The drawing under review shows one solid part. Ordinate dimensions are in mm from its lowest x, y, z. A direction names the side the tool comes from. Give positions to 0.01 mm unless a question says otherwise; leave off trailing zeros. Write each loop counter-clockwise with the first axis right and the second up, starting at its lowest first coordinate (ties: lowest second). Pieces come first, ordered by that corner, then holes.
Q1. We need section B-B (y = 11.25). Write out the cut boundary in (x, z), then the cut area to 3 significant figures.
Q2. Insertion check: P1, Ø4, axis at x = 5, y = 8, coming from the +Z side; P2, Ø1.5, axis at x = 5.5, y = 2.5, coming from the -Z side; P3, Ø3, axis at y = 7.5, z = 4.5, coming from the +X side. Each pin has a flat end and moves straight along its axis. Give the tip position at first contact, or say it passes through.
Q3. We need section A-A (y = 1.75). Write out the cut boundary in (x, z).
Q4. For line 1 (Y direction, x = 1.5, z = 2.5); line 2 (Y direction, x = 3.5, z = 2.5); line 3 (X direction, y = 14, z = 3.25), list the stretches that pass through material, from the lowest coordinate up.
Q5. Machinability: for the marked faces 1 and 2, which of the approach directions +Z, -Z, +X, -X, +Y, -Y give a long, thin tool a straight path to every point of the face, cutting with its end or side? Answer none if there is none.
Q6. Mouldability with a two-part tool opening along Z and no side actions: class the marked faces 3, 4, 5 and 6 as released by +Z, released by -Z, zero draft, split by the parting line, or undercut.
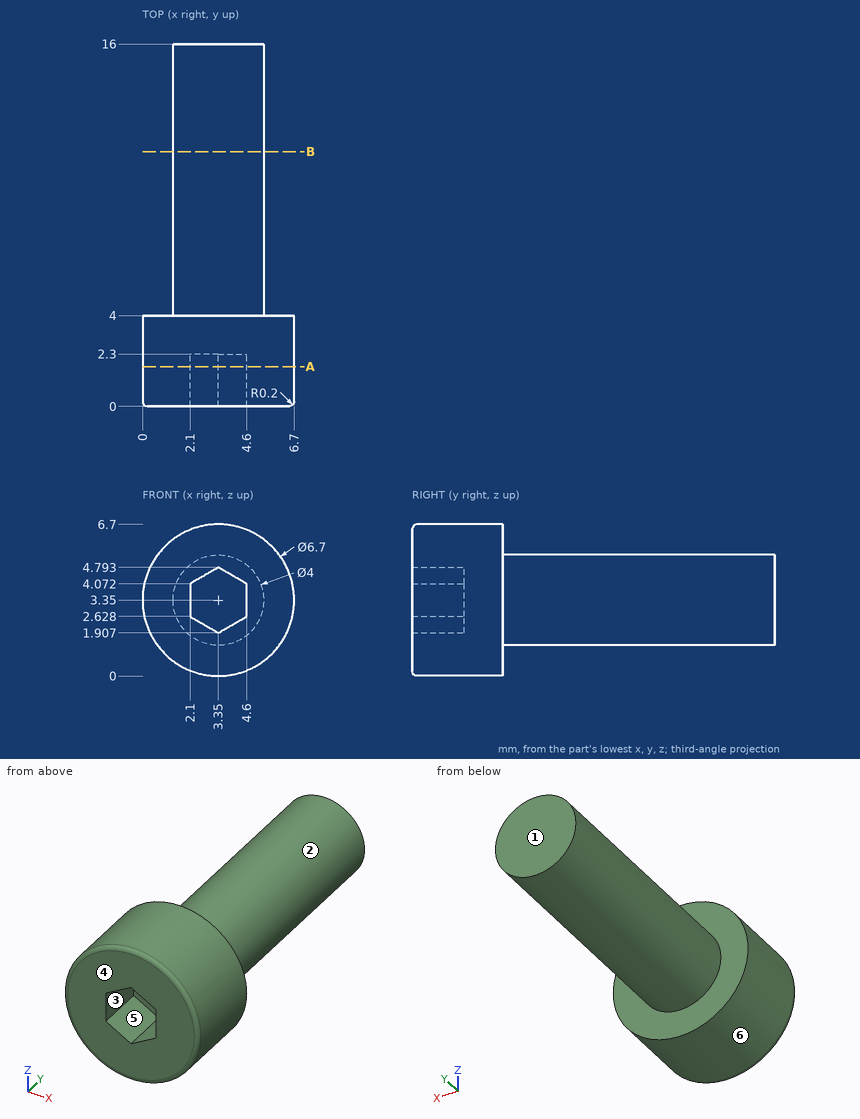
Computed:
1. outline: circle Ø4 at (3.35, 3.35)
1. area: 12.6 mm2
2. P1: stops at z = 5.35
2. P2: stops at z = 0.31
2. P3: stops at x = 5.35
3. outline: circle Ø6.7 at (3.35, 3.35); hole (2.1, 2.63) - (3.35, 1.91) - (4.6, 2.63) - (4.6, 4.07) - (3.35, 4.79) - (2.1, 4.07) - close
4. line 1: y = 0 to 4
4. line 2: y = 2.3 to 16
4. line 3: x = 1.35 to 5.35
5. face 1: +Z, -Z, +X, -X, +Y
5. face 2: +Y
6. face 3: undercut
6. face 4: zero draft
6. face 5: undercut
6. face 6: split by the parting line
